The model under review builds one solid part; all positions refer to its coordinate system, in mm. Face numbers are marked on the shaded views. A direction names the side the tool comes from. Round coordinates to 2 decimals unless told otherwise and drop trailing zeros. Order: outer loops, then holes, each group sorted by start corner. A loop starts at its lowest first (then second) coordinate and runs counter-clockwise, first axis right, second up. Notation, with made-up numbers: (28, 25) -> (32, 25) arc R31 ccw to (32, 63) -> close; hole circle Ø9 at (6, 67.25). An arc over 180 degrees is marked (long way). Use a Markdown table: item, result. Add a question column.
```python
from build123d import *

# Parameters (mm, degrees)
SKETCH2_W           = 64
SKETCH2_H           = 32
BOSS_EXTRUDE1_DEPTH = 5
SKETCH3_W           = 64
SKETCH3_H           = 10
BOSS_EXTRUDE2_DEPTH = 36
SKETCH4_W           = 64
SKETCH4_H           = 22
BOSS_EXTRUDE3_DEPTH = 10
BOSS_EXTRUDE4_DEPTH = 22
CUT_EXTRUDE1_DEPTH  = 33
SKETCH7_R           = 6
CUT_EXTRUDE2_DEPTH  = 24
LPATTERN1_COUNT     = 2
LPATTERN1_PITCH     = 16
FILLET1_R           = 3


with BuildPart() as part:
    # Sketch2 → Boss-Extrude1 (new body, symmetric)
    with BuildSketch(Plane(origin=(0, 0, 0), x_dir=(1, 0, 0), z_dir=(0, 1, 0))):
        Rectangle(SKETCH2_W, SKETCH2_H)
    extrude(amount=BOSS_EXTRUDE1_DEPTH, both=True)

    # Sketch3 → Boss-Extrude2 (add)
    with BuildSketch(Plane(origin=(0, 5, 0), x_dir=(1, 0, 0), z_dir=(0, 1, 0))):
        with Locations((0, 11)):
            Rectangle(SKETCH3_W, SKETCH3_H)
    extrude(amount=BOSS_EXTRUDE2_DEPTH)

    # Sketch4 → Boss-Extrude3 (add)
    with BuildSketch(Plane(origin=(0, 5, 0), x_dir=(1, 0, 0), z_dir=(0, 1, 0))):
        with Locations((0, -5)):
            Rectangle(SKETCH4_W, SKETCH4_H)
    extrude(amount=BOSS_EXTRUDE3_DEPTH)

    # Sketch5 → Boss-Extrude4 (add)
    with BuildSketch(Plane.XY.offset(16)):
        with BuildLine():
            Line((-27.5, 15), (27.5, 15))
            Line((27.5, 15), (12.8, 34.6))
            ThreePointArc((12.8, 34.6), (0, 41), (-12.8, 34.6))
            Line((-12.8, 34.6), (-27.5, 15))
        make_face()
    extrude(amount=-BOSS_EXTRUDE4_DEPTH)

    # Sketch6 → Cut-Extrude1 (cut)
    with BuildSketch(Plane.XY.offset(16)):
        Polygon((-32, 5), (-32, -5), (32, -5), (32, 5), (8, 5), (8, -4), (-8, -4), (-8, 5), align=None)
    extrude(amount=-CUT_EXTRUDE1_DEPTH, mode=Mode.SUBTRACT)

    # Sketch7 → Cut-Extrude2 (cut)
    with BuildSketch(Plane.XY.offset(16)):
        with Locations((0, 26.35)):
            Circle(SKETCH7_R)
    extrude(amount=-CUT_EXTRUDE2_DEPTH, mode=Mode.SUBTRACT)

    # Sketch10 → Cut-Revolve2 (revolve, cut)
    with BuildSketch(Plane.XY.offset(8)):
        Polygon((0, -4), (0, 13), (3, 12), (3, -4), align=None)
    cut_revolve2 = revolve(axis=Axis((0, -4, 8), (0, 1, 0)), mode=Mode.SUBTRACT)

    # LPattern1: Cut-Revolve2 ×2
    with Locations(*[(0, 0, -i * LPATTERN1_PITCH) for i in range(1, LPATTERN1_COUNT)]):
        add(cut_revolve2, mode=Mode.SUBTRACT)

    # Sketch15 → Cut-Revolve4 (revolve, cut)
    with BuildSketch(Plane(origin=(0, 0, 4), x_dir=(-1, 0, 0), z_dir=(0, 0, -1))):
        Polygon((-0.003619483, 30.011523803), (0, 41), (4.996380517, 41.011523803), (4.996380517, 38.011523803), (2.996380517, 38.011523803), (2.996380517, 31.011523803), align=None)
    revolve(axis=Axis((0.003619483, 30.011523803, 4), (-0.000329389, 0.999999946, 0)), mode=Mode.SUBTRACT)

    # Fillet1
    fillet1_edges = [part.edges().sort_by_distance(p)[0] for p in [
        (27.5, 15, 5),
        (-27.5, 15, 5),
    ]]
    fillet(fillet1_edges, radius=FILLET1_R)


solid = part.part
```
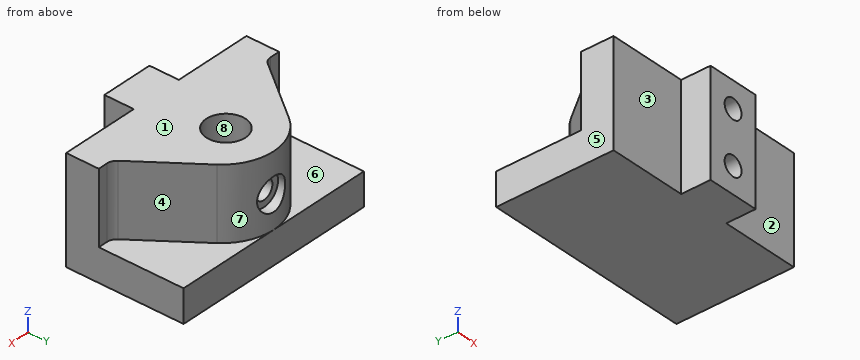
Q1. To check wall thickness, follow line 1 along X through (y, z) = (2, -8); line 2 along Z through (x, y) = (0, 2.5); line 3 along X through (y, z) = (7, -8). State the ranges of each line that lie inside material, in increasing order.
Q2. Add section C-C, the plane x = 10. Give the boundary of the cut face in (y, z), then the cut area to 3 significant figures.
Q3. For the marked faces 1, 2, 3 and 4, list the 3-axis set-ups (+Z, -Z, +X, -X, +Y, -Y) from which the entire face can be reached by the end or side of a thin tool; tool diameter is ignored.
Q4. Add section B-B, the plane y = -1. Give the boundary of the cut face in (x, z), then the cut area to 3 significant figures.
Q5. Add section D-D, the plane y = 26.35. Give the boundary of the cut face in (x, z).
Q6. Add section A-A, the plane z = -2.5. Give the boundary of the cut face in (x, y).
Q7. For pin 1 (10 mm diameter, centred on x = 23.5, z = 8, fed in from +Y); pin 2 (6 mm diameter, centred on x = 1.5, y = 25.5, fed in from +Z); pin 3 (3.5 mm diameter, centred on x = -30, z = 2, fed in from +Y), all flat-tipped, find the tip position at first contact; note any pin that passes through.
Q8. Draft analysis for pull direction X (two halves, no side actions). For the marked faces 5, 6, 7 and 8, state which applies: released by +X, released by -X, zero draft, split by the parting line, or undercut.
Return value:
| question | item | result |
|---|---|---|
| 1 | line 1 | -8 to -3, 3 to 8 |
| 1 | line 2 | -16 to -11, -5 to 5, 11 to 16 |
| 1 | line 3 | -32 to -3, 3 to 32 |
| 2 | outline | (5, -16) -> (41, -16) -> (41, -6) -> (37.49, -6) -> (37.49, 16) -> (5, 16) -> close |
| 2 | area | 1,070 mm² |
| 3 | face 1 | +Z, +X, -X, +Y, -Y |
| 3 | face 2 | +Z, -Z, +X, -Y |
| 3 | face 3 | +Z, -Z, -X, -Y |
| 3 | face 4 | +Z, +X, +Y |
| 4 | outline | (-8, -16) -> (8, -16) -> (8, 16) -> (-8, 16) -> close; hole circle Ø6 at (0, -8); hole circle Ø6 at (0, 8) |
| 4 | area | 455 mm² |
| 5 | outline | (-32, -16) -> (32, -16) -> (32, -6) -> (18.99, -6) -> (18.99, 16) -> (6, 16) -> (6, -8) -> (-6, -8) -> (-6, 16) -> (-18.99, 16) -> (-18.99, -6) -> (-32, -6) -> close |
| 6 | outline | (-32, 5) -> (-8, 5) -> (-8, -4) -> (8, -4) -> (8, 5) -> (32, 5) -> (32, 15) -> (29, 15) arc R3 cw to (26.6, 16.2) -> (12.8, 34.6) arc R16 ccw to (-12.8, 34.6) -> (-26.6, 16.2) arc R3 cw to (-29, 15) -> (-32, 15) -> close; hole circle Ø12 at (0, 26.35) |
| 7 | pin 1 | y = 27 |
| 7 | pin 2 | z = -8 |
| 7 | pin 3 | y = 15.1 |
| 8 | face 5 | released by -X |
| 8 | face 6 | zero draft |
| 8 | face 7 | split by the parting line |
| 8 | face 8 | undercut |
